```python
from build123d import *

# Parameters (mm, degrees)
BOSS_EXTRUDE1_DEPTH      = 13.57
BOSS_EXTRUDE3_DEPTH      = 3.5
BOSS_EXTRUDE4_DEPTH      = 26
BOSS_EXTRUDE4_DEPTH_BACK = 27
CUT_EXTRUDE1_DEPTH       = 45.729836908
CUT_EXTRUDE1_DEPTH_BACK  = 45.729836908
CUT_EXTRUDE2_DEPTH       = 46.64535365
CUT_EXTRUDE2_DEPTH_BACK  = 46.64535365
BOSS_EXTRUDE5_DEPTH      = 6
FILLET1_R                = 10
SKETCH8_R                = 2.15
CUT_EXTRUDE3_DEPTH       = 68.384074457
SKETCH8_4_R              = 3
SKETCH8_4_R_2            = 2.15
CUT_EXTRUDE4_DEPTH       = 3


with BuildPart() as part:
    # Sketch1 → Boss-Extrude1 (new body)
    with BuildSketch(Plane(origin=(0, 0, 0), x_dir=(1, 0, 0), z_dir=(0, 1, 0))):
        with BuildLine():
            Line((20, 7.5), (-20, 7.5))
            ThreePointArc((-20, 7.5), (-27.5, 0), (-20, -7.5))
            Line((-20, -7.5), (20, -7.5))
            ThreePointArc((20, -7.5), (27.5, 0), (20, 7.5))
        make_face()
    extrude(amount=BOSS_EXTRUDE1_DEPTH)

    # Sketch3 → Boss-Extrude3 (add)
    with BuildSketch(Plane(origin=(0, 13.57, 0), x_dir=(-1, 0, 0), z_dir=(0, -1, 0))):
        with BuildLine():
            Line((-19.549061387, 7.5), (19.549061387, 7.5))
            Line((19.549061387, 7.5), (12.499372909, 24.519453536))
            ThreePointArc((12.499372909, 24.519453536), (0, 12.144660941), (-12.499372909, 24.519453536))
            Line((-12.499372909, 24.519453536), (-19.549061387, 7.5))
        make_face()
        with BuildLine():
            ThreePointArc((-12.499372909, 24.519453536), (0, 12.144660941), (12.499372909, 24.519453536))
            Line((12.499372909, 24.519453536), (8.749856339, 33.57158729))
            ThreePointArc((8.749856339, 33.57158729), (8.625750618, 33.691562414), (8.5, 33.809812331))
            Line((8.5, 33.809812331), (8.5, 24.644660941))
            ThreePointArc((8.5, 24.644660941), (0, 16.144660941), (-8.5, 24.644660941))
            Line((-8.5, 24.644660941), (-8.5, 33.809812331))
            ThreePointArc((-8.5, 33.809812331), (-8.625750618, 33.691562414), (-8.749856339, 33.57158729))
            Line((-8.749856339, 33.57158729), (-12.499372909, 24.519453536))
        make_face()
    extrude(amount=BOSS_EXTRUDE3_DEPTH)

    # Sketch4 → Boss-Extrude4 (add, two sides: drawn at the far end of the back side and taken through both)
    with BuildSketch(Plane(origin=(0, 0, 0), x_dir=(0, 0, -1), z_dir=(1, 0, 0)).offset(-BOSS_EXTRUDE4_DEPTH_BACK)):
        Polygon((7.5, 10.07), (7.5, 7.17), (17.5, 10.07), align=None)
    extrude(amount=BOSS_EXTRUDE4_DEPTH + BOSS_EXTRUDE4_DEPTH_BACK)

    # Sketch5 → Cut-Extrude1 (cut, two sides: drawn at the far end of the back side and taken through both)
    with BuildSketch(Plane(origin=(0, 10.07, 0), x_dir=(1, 0, 0), z_dir=(0, 1, 0)).offset(-CUT_EXTRUDE1_DEPTH_BACK)):
        Polygon((-19.549061387, 7.5), (-15.406925764, 17.5), (-27, 17.5), (-27, 7.5), (-20, 7.5), align=None)
        Polygon((15.406925764, 17.5), (19.549061387, 7.5), (20, 7.5), (26, 7.5), (26, 17.5), align=None)
        with BuildLine():
            Line((4.604760585, 17.5), (-4.604760585, 17.5))
            ThreePointArc((-4.604760585, 17.5), (0, 16.144660941), (4.604760585, 17.5))
        make_face()
    extrude(amount=CUT_EXTRUDE1_DEPTH + CUT_EXTRUDE1_DEPTH_BACK, mode=Mode.SUBTRACT)

    # Sketch6 → Cut-Extrude2 (cut, two sides: drawn at the far end of the back side and taken through both)
    with BuildSketch(Plane(origin=(0, 0, 0), x_dir=(0, 0, -1), z_dir=(1, 0, 0)).offset(-CUT_EXTRUDE2_DEPTH_BACK)):
        Polygon((32.504181683, 4.538254004), (33.809812331, 6.646903952), (33.809812331, 13.57), (25, 10.07), align=None)
    extrude(amount=CUT_EXTRUDE2_DEPTH + CUT_EXTRUDE2_DEPTH_BACK, mode=Mode.SUBTRACT)

    # Sketch7 → Boss-Extrude5 (add)
    with BuildSketch(Plane(origin=(0, 0, 0), x_dir=(1, 0, 0), z_dir=(0, 1, 0))):
        with BuildLine():
            Line((57.794508063, 19.700472411), (49.648476863, 33.809812331))
            ThreePointArc((49.648476863, 33.809812331), (0, 7.5), (-49.648476863, 33.809812331))
            Line((-49.648476863, 33.809812331), (-57.794508063, 19.700472411))
            ThreePointArc((-57.794508063, 19.700472411), (-31.93771633, -0.360019714), (-3.1e-07, -7.5))
            ThreePointArc((-3.1e-07, -7.5), (31.93771605, -0.360019846), (57.794508063, 19.700472411))
        make_face()
    extrude(amount=BOSS_EXTRUDE5_DEPTH)

    # Fillet1
    # the kernel refuses this fillet: 10 mm, written as the material it takes off along each edge
    with BuildSketch(Plane(origin=(-38.192037625, 6, -53.652947164), x_dir=(0.8660254037844376, 0, 0.5000000000000019), z_dir=(-0.5000000000000019, 0, 0.8660254037844376))) as fillet1_piece_1:
        with BuildLine():
            CenterArc((9.16515139, -10), FILLET1_R, 90, 66.421821522)
            Line((0, -6), (-0.183303028, -5.92))
            ThreePointArc((-0.183303028, -5.92), (-0.2, -3), (-0.2, 0))
            Line((-0.2, 0), (0, 0.2))
            Line((0, 0.2), (9.16515139, 0.2))
            Line((9.16515139, 0.2), (9.16515139, 0))
        make_face()
    extrude(amount=62.117819351, mode=Mode.SUBTRACT)
    with BuildSketch(Plane(origin=(69.250947301, 6, 0.142662422), x_dir=(0, -1, 0), z_dir=(-0.5000000000000019, 0, -0.8660254037844376))) as fillet1_piece_2:
        with BuildLine():
            CenterArc((10, 9.16515139), FILLET1_R, 180, 66.421821522)
            Line((0, 9.16515139), (-0.2, 9.16515139))
            Line((-0.2, 9.16515139), (-0.2, 0))
            Line((-0.2, 0), (0, -0.2))
            ThreePointArc((0, -0.2), (3, -0.2), (5.92, -0.183303028))
            Line((5.92, -0.183303028), (6, 0))
        make_face()
    extrude(amount=62.117819351, mode=Mode.SUBTRACT)

    # Sketch8 → Cut-Extrude3 (cut, through all)
    with BuildSketch(Plane(origin=(0, 6, 0), x_dir=(1, 0, 0), z_dir=(0, 1, 0))):
        with Locations(Location((37.064396977, 11.087510982, 0), (0, 0, 270))):
            Circle(SKETCH8_R)
        with Locations(Location((-37.064396977, 11.087510982, 0), (0, 0, 270))):
            Circle(SKETCH8_R)
    extrude(amount=-CUT_EXTRUDE3_DEPTH, mode=Mode.SUBTRACT)

    # Sketch8<4> → Cut-Extrude4 (cut)
    # profile 1 of 2: a face of its own
    with BuildSketch(Plane(origin=(0, 6, 0), x_dir=(1, 0, 0), z_dir=(0, 1, 0))):
        with Locations(Location((37.064396977, 11.087510982, 0), (0, 0, 270))):
            Circle(SKETCH8_4_R)
        with Locations(Location((37.064396977, 11.087510982, 0), (0, 0, 270))):
            Circle(SKETCH8_4_R_2, mode=Mode.SUBTRACT)
    # profile 2 of 2: a face of its own
    with BuildSketch(Plane(origin=(0, 6, 0), x_dir=(1, 0, 0), z_dir=(0, 1, 0))):
        with Locations(Location((-37.064396977, 11.087510982, 0), (0, 0, 90))):
            Circle(SKETCH8_4_R)
        with Locations(Location((-37.064396977, 11.087510982, 0), (0, 0, 270))):
            Circle(SKETCH8_4_R_2, mode=Mode.SUBTRACT)
    extrude(amount=-CUT_EXTRUDE4_DEPTH, mode=Mode.SUBTRACT)


solid = part.part
```
Model file for the job. Use its own axes, mm. A direction names the side the tool comes from. Round coordinates to 2 decimals unless told otherwise and drop trailing zeros. Write each loop counter-clockwise with the first axis right and the second up, starting at its lowest first coordinate (ties: lowest second). Pieces come first, ordered by that corner, then holes. Notation, with made-up numbers: M 78.5,87 L 109.5,87 A10 ccw 109.5,103 Z; hole C 25.5,-17.75 d10. An arc over 180 degrees is marked long. Put each result on its own line as item: value.
Item 1: Mould opens along X. For faces 5 (the cylindrical face through (43.65, 2.96, -6.51)), 6 (the flat face through (10, 10.07, -20)), 7 (the cylindrical face through (34.403, 4.521, -9.703)) say: +X half, -X half, draft (parallel to the pull), parting line (faces both ways), or undercut.
Responses:
face 5: +X half
face 6: draft
face 7: undercut
Item 2: Tool access for faces 1 (the cylindrical face through (26.99, 8.2, 2.72)), 2 (the flat face through (-11, 10.07, -20)), 3 (the flat face through (-8.5, 12, -28)), 4 (the cylindrical face through (-34.136, 4.521, -10.437)): list every direction of +Z, -Z, +X, -X, +Y, -Y with a clear straight run to the whole face (end or side of a thin tool).
Responses:
face 1: +X, +Y
face 2: -Z, +X, -X, -Y
face 3: -Z, +Y, -Y
face 4: +Y
Item 3: Probe L1, parallel to Y at x = 43.5, z = -10; L2, parallel to X at y = 0.5, z = -26; L3, parallel to X at y = 5, z = -23. List the from-to ranges inside material, lowest first. Write a range as from..to.
Responses:
L1: 0..6
L2: -53.89..-43.33, 43.33..53.89
L3: -50.34..-40.25, 40.25..50.34
Item 4: Cut at D-D (y = 12.25). List the corners of the cut face in (x, z), and give its area (3 significant figures).
Responses:
outline: M -20,-7.5 L -19.55,-7.5 L -10.03,-30.49 L -8.5,-30.49 L -8.5,-24.64 A8.5 cw 8.5,-24.64 L 8.5,-30.49 L 10.03,-30.49 L 19.55,-7.5 L 20,-7.5 A7.5 ccw 20,7.5 L -20,7.5 A7.5 ccw Z
area: 1,240 mm²
Item 5: Flat gauge pins, fed straight in: P1, Ø8, axis at x = 43, z = -25.5, coming from the +Y side; P2, Ø3, axis at y = 12, z = -27, coming from the +X side; P3, Ø6, axis at x = -39.5, z = -27.5, coming from the +Y side; P4, Ø6, axis at x = -3, y = 10, coming from the -Z side. Where does each tip first touch, or does it go through?
Responses:
P1: y = 6
P2: x = 12.09
P3: through
P4: z = -18.62
Item 6: Cut at C-C (z = 0). List the corners of the cut face in (x, y).
Responses:
outline: M -32.69,0 L 32.69,0 L 32.69,6 L 27.5,6 L 27.5,13.57 L -27.5,13.57 L -27.5,6 L -32.69,6 Z
Item 7: Cut at A-A (y = 1.75). List the corners of the cut face in (x, z), and give its area (3 significant figures).
Responses:
outline: M -57.12,-18.9 L -49.03,-32.91 A60 cw 49.03,-32.91 L 57.12,-18.9 A75 ccw 27.09,2.44 A7.5 ccw 20,7.5 L -20,7.5 A7.5 ccw -27.09,2.44 A75 ccw Z; hole C -37.06,-11.09 d4.3; hole C 37.06,-11.09 d4.3
area: 1,880 mm²
Item 8: Cut at B-B (x = -21). List the corners of the cut face in (y, z), and give its area (3 significant figures).
Responses:
outline: M 0,-11.3 L 6,-11.3 L 6,-7.43 L 13.57,-7.43 L 13.57,7.43 L 0,7.43 Z
area: 225 mm²
